from build123d import *

# Parameters (mm, degrees)
SKETCH_R     = 25
PAD_DEPTH    = 8
SKETCH001_R  = 2.5
PAD001_DEPTH = 4


with BuildPart() as part:
    # Sketch → Pad (new body)
    with BuildSketch(Plane.XZ):
        Circle(SKETCH_R)
    extrude(amount=PAD_DEPTH)

    # Sketch001 → Pad001 (join, symmetric)
    with BuildSketch(Plane.YZ):
        Polygon((18.95327, 22.469796), (34.996391, 47.819712), (38.451828, 18.019377), (68.273913, 21.281774), (47.129503, 0), (68.273913, -21.281774), (38.451828, -18.019377), (34.996391, -47.819712), (18.95327, -22.469796), (-6.5, -38.348432), (3.31664, -10), (0, -8.827391), (0, 8.827391), (3.31664, 10), (-6.5, 38.348432), align=None)
        with Locations((16.276457, 7.884052)):
            Circle(SKETCH001_R, mode=Mode.SUBTRACT)
        with Locations((31.440147, 7.884052)):
            Circle(SKETCH001_R, mode=Mode.SUBTRACT)
        with BuildLine():
            ThreePointArc((15.563428, -7.94964), (24.081854, -14.045087), (32.600279, -7.94964))
            ThreePointArc((15.563428, -7.94964), (24.081854, -11.301611), (32.600279, -7.94964))
        make_face(mode=Mode.SUBTRACT)
    extrude(amount=PAD001_DEPTH, both=True)


solid = part.part
The listing builds one solid part. Answer for the finished solid, in the listing's coordinates (mm). A direction names the side the tool comes from. Round coordinates to 2 decimals unless told otherwise and drop trailing zeros. Order: outer loops, then holes, each group sorted by start corner. A loop starts at its lowest first (then second) coordinate and runs counter-clockwise, first axis right, second up. Notation, with made-up numbers: M 68.25,14.5 L 81.25,14.5 A23 ccw 81.25,41.5 Z; hole C 63.5,25.5 d8. An arc over 180 degrees is marked long. Answer in a Markdown table with one row per item. Add a question column.
1) Consider line 1 along X through (y, z) = (58, 17); line 2 along Y through (x, z) = (-19, -6); line 3 along Y through (x, z) = (1, -25.5). Determine where each line is inside the solid, lowest interval first. Write a range as from..to.
2) Flat-ended cylindrical pins translate along their axes: pin 1 Ø5 at (y, z) = (16, 30) entering from -X; pin 2 Ø3 at (x, y) = (2.5, 51.5) entering from +Z; pin 3 Ø10 at (x, z) = (3.5, 38) entering from -Y; pin 4 Ø10 at (x, y) = (2.5, 20) entering from -Z. Find the tip coordinate at first contact, or state that the pin passes through.
3) Determine the mould class of faces 5 (the face through (0, -8, 0)), 6 (the face through (-0.06, 29.46, 6.36)), 7 (the face through (0.056, 53.572, -19.673)) for opening direction Z: pulls with the +Z half, pulls with the -Z half, needs draft (parallel to the pull), parting line crosses it, or undercut.
4) The part is cut by section C-C on x = 0. Determine the outline of the cut face in (y, z).
5) Which of the six approach directions +Z, -Z, +X, -X, +Y, -Y give full straight-line access (tool end or side, diameter ignored) to faces 1 (the face through (0.056, 26.863, 34.967)), 2 (the face through (0.1, 6.4, -30.3)), 3 (the face through (0.06, 57.85, 10.79)), 4 (the face through (-0.056, 14.293, 6.363))?
6) The part is cut by section A-A on y = 60. Determine the outline of the cut face in (x, z).
7) The part is cut by section D-D on x = -20.5. Determine the outline of the cut face in (y, z).
8) The part is cut by section B-B on z = -32. Determine the outline of the cut face in (x, y), plus the area to 3 significant figures.
Findings below:
| question | item | result |
|---|---|---|
| 1 | line 1 | x = -4..4 |
| 1 | line 2 | y = -8..0 |
| 1 | line 3 | y = -2.05..14.1, 20.87..37.58 |
| 2 | pin 1 | passes through |
| 2 | pin 2 | stops at z = 19.61 |
| 2 | pin 3 | stops at y = -6.5 |
| 2 | pin 4 | stops at z = -32.02 |
| 3 | face 5 | needs draft |
| 3 | face 6 | undercut |
| 3 | face 7 | pulls with the -Z half |
| 4 | outline | M -8,-25 L -1.88,-25 L -6.5,-38.35 L 18.95,-22.47 L 35,-47.82 L 38.45,-18.02 L 68.27,-21.28 L 47.13,0 L 68.27,21.28 L 38.45,18.02 L 35,47.82 L 18.95,22.47 L -6.5,38.35 L -1.88,25 L -8,25 Z; hole M 0,-19.58 L 3.32,-10 L 0,-8.83 Z; hole M 0,8.83 L 3.32,10 L 0,19.58 Z; hole C 16.28,7.88 d5; hole M 15.56,-7.95 A9 ccw 32.6,-7.95 A12.5 cw Z; hole C 31.44,7.88 d5 |
| 5 | face 1 | +Z, +X, -X |
| 5 | face 2 | -Z, +X, -X |
| 5 | face 3 | +X, -X, +Y |
| 5 | face 4 | +X, -X |
| 6 | outline | M -4,-20.38 L 4,-20.38 L 4,-12.95 L -4,-12.95 Z; M -4,12.95 L 4,12.95 L 4,20.38 L -4,20.38 Z |
| 7 | outline | M -8,-14.31 L 0,-14.31 L 0,14.31 L -8,14.31 Z |
| 8 | outline | M -4,-4.3 L 4,-4.3 L 4,3.68 L -4,3.68 Z; M -4,24.98 L 4,24.98 L 4,36.83 L -4,36.83 Z |
| 8 | area | 159 mm² |
